Geometry check sheet. Reference: the model listing, model coordinates, mm. Face numbers are marked on the shaded views. A direction names the side the tool comes from. Give positions to 0.01 mm unless a question says otherwise; leave off trailing zeros. Loops run counter-clockwise (first coordinate to the right, second up) from the corner with the lowest first, then second, coordinate; pieces in that order, holes last. Notation, with made-up numbers: (-26.75, 72) - (-8.75, 72) arc R22 ccw to (-8.75, 84) - close; hole circle Ø1 at (88, 43). An arc over 180 degrees is marked (long way). Use a Markdown table: item, result. Add a question column.
1. Cross-section at C-C on y = 15. Enter the section's corners in (x, z), and give its area (3 significant figures).
2. Draft check along X on the marked faces 1, 2 and 3. Enter one of: pulls with the +X half, pulls with the -X half, needs draft (parallel to the pull), parting line crosses it, or undercut.
3. Set-up check for the marked faces 4, 5 and 6: record each of +Z, -Z, +X, -X, +Y, -Y from which the full face is reachable in a straight line by a thin tool's end or side.
4. Cross-section at B-B on z = 0. Enter the section's corners in (x, y).
5. Cross-section at D-D on y = 26. Enter the section's corners in (x, z), and give its area (3 significant figures).
6. Depth check by flat-ended pin: P1, Ø3, axis at x = 51.5, z = 10.5, coming from the -Y side; P2, Ø2, axis at y = 16, z = 11, coming from the +X side; P3, Ø1, axis at x = 27, y = 17.5, coming from the +Z side. Enter the tip coordinate at first touch or a pass-through.
7. Cross-section at A-A on x = -2.5. Enter the section's corners in (y, z), and give its area (3 significant figures).
8. Material ranges on L1, parallel to X at y = 25, z = 1; L2, parallel to Z at x = -3, y = 9.25; L3, parallel to X at y = 17.25, z = -3.5, recorded low to high.
from build123d import *

# Parameters (mm, degrees)
BOSS_EXTRUDE1_DEPTH = 30
SKETCH2_R           = 7.5
BOSS_EXTRUDE2_DEPTH = 50


with BuildPart() as part:
    # Sketch1 → Boss-Extrude1 (new body)
    with BuildSketch(Plane(origin=(0, 0, 0), x_dir=(1, 0, 0), z_dir=(0, 1, 0))):
        with BuildLine():
            Line((-10, 20), (10, 20))
            ThreePointArc((10, 20), (13.535533906, 18.535533906), (15, 15))
            Line((15, 15), (15, -15))
            ThreePointArc((15, -15), (13.535533906, -18.535533906), (10, -20))
            Line((10, -20), (-10, -20))
            ThreePointArc((-10, -20), (-17.071067812, -17.071067812), (-20, -10))
            Line((-20, -10), (-20, 10))
            ThreePointArc((-20, 10), (-17.071067812, 17.071067812), (-10, 20))
        make_face()
        with BuildLine():
            Line((-12.5, 5), (-12.5, -5))
            ThreePointArc((-12.5, -5), (-2.5, -15), (7.5, -5))
            Line((7.5, -5), (7.5, 5))
            ThreePointArc((7.5, 5), (-2.5, 15), (-12.5, 5))
        make_face(mode=Mode.SUBTRACT)
    extrude(amount=BOSS_EXTRUDE1_DEPTH)

    # Sketch2 → Boss-Extrude2 (add)
    with BuildSketch(Plane(origin=(15, 0, 0), x_dir=(0, 0, -1), z_dir=(1, 0, 0))):
        with Locations(Location((0, 15, 0), (0, 0, 180))):
            Circle(SKETCH2_R)
    extrude(amount=BOSS_EXTRUDE2_DEPTH)


solid = part.part
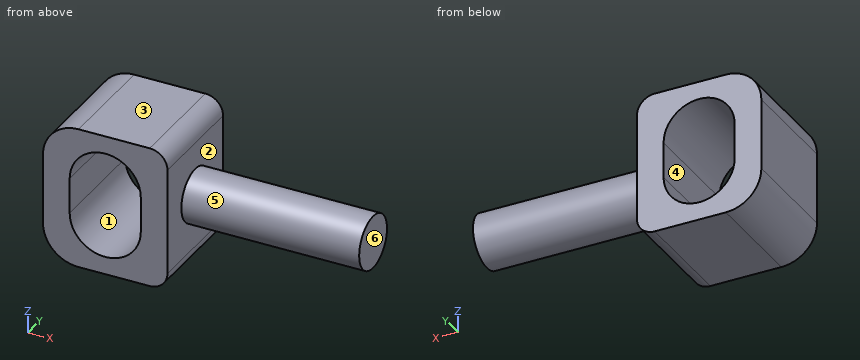
Values found:
| question | item | result |
|---|---|---|
| 1 | outline | (-20, -10) arc R10 ccw to (-10, -20) - (10, -20) arc R5 ccw to (15, -15) - (15, -7.5) - (65, -7.5) - (65, 7.5) - (15, 7.5) - (15, 15) arc R5 ccw to (10, 20) - (-10, 20) arc R10 ccw to (-20, 10) - close; hole (-12.5, -5) arc R10 ccw to (7.5, -5) - (7.5, 5) arc R10 ccw to (-12.5, 5) - close |
| 1 | area | 1,580 mm2 |
| 2 | face 1 | undercut |
| 2 | face 2 | pulls with the +X half |
| 2 | face 3 | needs draft |
| 3 | face 4 | +Y, -Y |
| 3 | face 5 | +X |
| 3 | face 6 | +Z, -Z, +X, +Y, -Y |
| 4 | outline | (-20, 0) - (-12.5, 0) - (-12.5, 30) - (-20, 30) - close; (7.5, 0) - (15, 0) - (15, 7.5) - (65, 7.5) - (65, 22.5) - (15, 22.5) - (15, 30) - (7.5, 30) - close |
| 5 | outline | (-20, -10) arc R10 ccw to (-10, -20) - (10, -20) arc R5 ccw to (15, -15) - (15, 15) arc R5 ccw to (10, 20) - (-10, 20) arc R10 ccw to (-20, 10) - close; hole (-12.5, -5) arc R10 ccw to (7.5, -5) - (7.5, 5) arc R10 ccw to (-12.5, 5) - close |
| 5 | area | 832 mm2 |
| 6 | P1 | passes through |
| 6 | P2 | stops at x = 15 |
| 6 | P3 | stops at z = 7.23 |
| 7 | outline | (0, -20) - (30, -20) - (30, -15) - (0, -15) - close; (0, 15) - (30, 15) - (30, 20) - (0, 20) - close |
| 7 | area | 300 mm2 |
| 8 | L1 | x = -20 to -12.5, 7.5 to 15 |
| 8 | L2 | z = -20 to -14.99, 14.99 to 20 |
| 8 | L3 | x = -20 to -12.5, 7.5 to 65 |
